Could you check a few things on this model? Use its own coordinates, in mm. A direction names the side the tool comes from. Round coordinates to 2 decimals unless told otherwise and drop trailing zeros. Loops run counter-clockwise (first coordinate to the right, second up) from the corner with the lowest first, then second, coordinate; pieces in that order, holes last. Notation, with made-up numbers: (44.25, -24) -> (89.25, -24) arc R18 cw to (89.25, -7) -> close; hole circle Ø2 at (4.5, -17.5). An arc over 180 degrees is marked (long way). Use CSV: the item, a comma, the result in double quotes. Start each with the question number.
```python
from build123d import *

# Parameters (mm, degrees)
F0_W        = 100.4
F0_H        = 81.6
F1_DEPTH    = 4.5
F2_T1_DEPTH = 125.6339057619
F2_T3_DEPTH = 106.8339057619
F3_T        = -2.54


# Not quite as in the source:
# - a fillet or chamfer that OpenCascade refuses, or shapes differently, is made with other operations: its cross-section is extruded or revolved along the edge and cut away or added


with BuildPart() as f1:
    # F0 (on Top) → F1 (new body)
    with BuildSketch(Plane.XY):
        with Locations((-0.9694248438, 10.5918823534)):
            Rectangle(F0_W, F0_H)
    extrude(amount=F1_DEPTH)

    # F2: fillet of radius 5.08 on 4 edges, made by hand

    # F2_s2 → F2_t1 (cut)
    with BuildSketch(Plane.YZ.offset(-63.7863777247)):
        with BuildLine():
            ThreePointArc((51.3918823534, 0), (49.7259295019, 3.2116223441), (46.345101201, 4.5))
            Line((46.345101201, 4.5), (51.3918823534, 4.5))
            Line((51.3918823534, 4.5), (51.3918823534, 0))
        make_face()
        with BuildLine():
            ThreePointArc((-30.2081176466, 0), (-28.5421647951, 3.2116223441), (-25.1613364942, 4.5))
            Line((-25.1613364942, 4.5), (-30.2081176466, 4.5))
            Line((-30.2081176466, 4.5), (-30.2081176466, 0))
        make_face()
    extrude(amount=F2_T1_DEPTH, mode=Mode.SUBTRACT)

    # F2_s4 → F2_t3 (cut)
    with BuildSketch(Plane.XZ.offset(-64.0088352343)):
        with BuildLine():
            ThreePointArc((-51.1694248438, 0), (-49.5034719923, 3.2116223441), (-46.1226436914, 4.5))
            Line((-46.1226436914, 4.5), (-51.1694248438, 4.5))
            Line((-51.1694248438, 4.5), (-51.1694248438, 0))
        make_face()
        with BuildLine():
            ThreePointArc((49.2305751562, 0), (47.5646223047, 3.2116223441), (44.1837940038, 4.5))
            Line((44.1837940038, 4.5), (49.2305751562, 4.5))
            Line((49.2305751562, 4.5), (49.2305751562, 0))
        make_face()
    extrude(amount=F2_T3_DEPTH, mode=Mode.SUBTRACT)

    # F3
    f3_openings = [f1.faces().sort_by_distance(p)[0] for p in [
        (-0.969425, 10.591882, 0),
    ]]
    offset(amount=F3_T, openings=f3_openings)


solid = f1.part
```
1. For faces 1 (the face through (-47.719, 11.127, 1.396)), 2 (the face through (-1.67, -28.58, 3.18)), which set-ups out of +Z, -Z, +X, -X, +Y, -Y let a thin tool reach every point of the face, with its end or its side?
2. We'd pull the mould along Y, two halves only. Please class faces 3 (the face through (45.78, 11.127, 1.396)), 4 (the face through (-1.67, 49.76, 3.18)), 5 (the face through (-5, -29, 0)): pulls with the +Y half, pulls with the -Y half, needs draft (parallel to the pull), parting line crosses it, or undercut.
3. Suppose I cut it at A-A (x = 3). List the corners of the cut face in (y, z) for me.
4. Suppose I cut it at C-C (z = 3.6). List the corners of the cut face in (x, y) for me.
5. If I drill on L1, parallel to Z at x = -3, y = -12; L2, parallel to X at y = -26, z = 1.1; L3, parallel to Y at x = -9, z = 1.7, over which ranges is the centre line in solid material (lowest first)?
6. Will these pins go through, and if not, where does the flat tip stop? pin 1 (21.5 mm diameter, centred on x = -12.5, y = 5, fed in from -Z); pin 2 (2 mm diameter, centred on y = 34.5, z = 1, fed in from +X).
7. Suppose I cut it at B-B (y = -22.5). List the corners of the cut face in (x, z) for me, then the cut area to 3 significant figures.
Geometry check:
1,face 1,"-Z"
1,face 2,"+Z, +X, -X, -Y"
2,face 3,"undercut"
2,face 4,"pulls with the +Y half"
2,face 5,"needs draft"
3,outline,"(-30.21, 0) -> (-27.63, 0) arc R2.54 cw to (-25.16, 1.96) -> (46.35, 1.96) arc R2.54 cw to (48.82, 0) -> (51.39, 0) arc R5.08 ccw to (46.35, 4.5) -> (-25.16, 4.5) arc R5.08 ccw to start"
4,outline,"(-49.01, -28.05) -> (47.07, -28.05) -> (47.07, 49.23) -> (-49.01, 49.23) -> close"
5,L1,"z = 1.96 to 4.5"
5,L2,"x = -50.92 to -48.03, 46.09 to 48.98"
5,L3,"y = -29.7 to -26.28, 47.46 to 50.88"
6,pin 1,"stops at z = 1.96"
6,pin 2,"stops at x = 49.23"
7,outline,"(-51.17, 0) -> (-48.6, 0) arc R2.54 cw to (-46.12, 1.96) -> (44.18, 1.96) arc R2.54 cw to (46.66, 0) -> (49.23, 0) arc R5.08 ccw to (44.18, 4.5) -> (-46.12, 4.5) arc R5.08 ccw to start"
7,area,"257 mm²"
